CAD build for the part. Positions are in the model's coordinates, mm. Face numbers are marked on the shaded views. A direction names the side the tool comes from. Coordinates: 2 decimals unless noted, no trailing zeros. Loops run counter-clockwise (first coordinate to the right, second up) from the corner with the lowest first, then second, coordinate; pieces in that order, holes last. Notation, with made-up numbers: (82, -35) -> (125, -35) arc R9 ccw to (125, -24) -> close; hole circle Ø11 at (-9.75, 87.25). An arc over 180 degrees is marked (long way). Answer as a JSON object with one key per item and string values. Group by question number.
from build123d import *

# Parameters (mm, degrees)
SKETCH1_W           = 163
SKETCH1_H           = 113
OUTERCUT_DEPTH      = 23
FILLET2_R           = 2.5
FILLET3_R           = 2.5
SKETCH2_W           = 155
SKETCH2_H           = 105
INNERCUT_DEPTH      = 20
BOSS_EXTRUDE5_DEPTH = 3


with BuildPart() as part:
    # Sketch1 → OuterCut (new body)
    with BuildSketch(Plane(origin=(0, 0, 0), x_dir=(1, 0, 0), z_dir=(0, 1, 0))):
        Rectangle(SKETCH1_W, SKETCH1_H)
    extrude(amount=OUTERCUT_DEPTH)

    # Fillet2
    fillet2_edges = [part.edges().sort_by_distance(p)[0] for p in [
        (81.5, 11.5, 56.5),
    ]]
    fillet(fillet2_edges, radius=FILLET2_R)

    # Fillet3
    fillet3_edges = [part.edges().sort_by_distance(p)[0] for p in [
        (-81.5, 11.5, 56.5),
        (-81.5, 11.5, -56.5),
        (81.5, 11.5, -56.5),
    ]]
    fillet(fillet3_edges, radius=FILLET3_R)

    # Sketch2 → InnerCut (cut)
    with BuildSketch(Plane(origin=(0, 23, 0), x_dir=(1, 0, 0), z_dir=(0, 1, 0))):
        Rectangle(SKETCH2_W, SKETCH2_H)
    extrude(amount=-INNERCUT_DEPTH, mode=Mode.SUBTRACT)

    # Sketch9 → Boss-Extrude5 (add)
    with BuildSketch(Plane(origin=(0, 23, 0), x_dir=(1, 0, 0), z_dir=(0, 1, 0))):
        with BuildLine():
            Line((58.5, -53.7), (61.5, -53.7))
            ThreePointArc((61.5, -53.7), (62.3, -54.5), (61.5, -55.3))
            Line((61.5, -55.3), (58.5, -55.3))
            ThreePointArc((58.5, -55.3), (57.7, -54.5), (58.5, -53.7))
        make_face()
        with BuildLine():
            Line((-61.5, -53.7), (-58.5, -53.7))
            ThreePointArc((-58.5, -53.7), (-57.7, -54.5), (-58.5, -55.3))
            Line((-58.5, -55.3), (-61.5, -55.3))
            ThreePointArc((-61.5, -55.3), (-62.3, -54.5), (-61.5, -53.7))
        make_face()
        with BuildLine():
            Line((-61.5, 55.3), (-58.5, 55.3))
            ThreePointArc((-58.5, 55.3), (-57.7, 54.5), (-58.5, 53.7))
            Line((-58.5, 53.7), (-61.5, 53.7))
            ThreePointArc((-61.5, 53.7), (-62.3, 54.5), (-61.5, 55.3))
        make_face()
        with BuildLine():
            Line((58.5, 55.3), (61.5, 55.3))
            ThreePointArc((61.5, 55.3), (62.3, 54.5), (61.5, 53.7))
            Line((61.5, 53.7), (58.5, 53.7))
            ThreePointArc((58.5, 53.7), (57.7, 54.5), (58.5, 55.3))
        make_face()
    extrude(amount=BOSS_EXTRUDE5_DEPTH)


solid = part.part
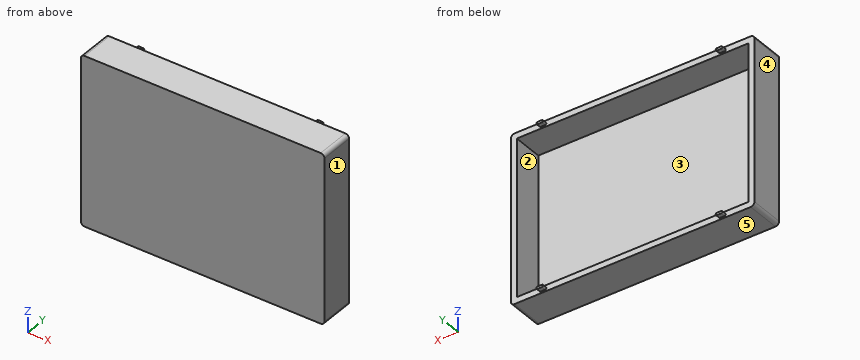
Item 1: Band-saw the part on B-B, the plane y = 17.5. List the corners of the cut face in (x, z).
Item 2: 3-axis set-ups, long thin cutter, end or side, ignore diameter. For the marked faces 1 and 2: which of +Z, -Z, +X, -X, +Y, -Y reach the whole face in a straight line?
Item 3: Flat gauge pins, fed straight in: P1, Ø3.5, axis at x = -60.5, y = 25, coming from the -Z side; P2, Ø1.5, axis at x = -10.5, z = -39.5, coming from the +Y side; P3, Ø0.9, axis at x = 60, y = 25, coming from the +Z side. Where does each tip first touch, or does it go through?
Item 4: Band-saw the part on C-C, the plane x = -7.5. List the corners of the cut face in (y, z), and give its area (3 significant figures).
Item 5: Band-saw the part on A-A, the plane z = 44.5. List the corners of the cut face in (x, y).
Item 6: Pull direction Z, two halves, no side cores. Call the marked faces 3, 4 and 5: +Z half, -Z half, draft (parallel to the pull), parting line (faces both ways), or undercut.
Item 7: Drill centre lines: L1, parallel to Z at x = 43, y = 9.5; L2, parallel to X at y = 14, z = 42; L3, parallel to Y at x = 20, z = -41. Where is each one in solid material? Low to high.
Reply:
{
 "1": {"outline": "(-81.5, -54) arc R2.5 ccw to (-79, -56.5) -> (79, -56.5) arc R2.5 ccw to (81.5, -54) -> (81.5, 54) arc R2.5 ccw to (79, 56.5) -> (-79, 56.5) arc R2.5 ccw to (-81.5, 54) -> close; hole (-77.5, -52.5) -> (77.5, -52.5) -> (77.5, 52.5) -> (-77.5, 52.5) -> close"},
 "2": {"face 1": "+Z, -Z, +X, +Y, -Y", "face 2": "+Y"},
 "3": {"P1": "z = -55.3", "P2": "y = 3", "P3": "z = 55.3"},
 "4": {"outline": "(0, -56.5) -> (23, -56.5) -> (23, -52.5) -> (3, -52.5) -> (3, 52.5) -> (23, 52.5) -> (23, 56.5) -> (0, 56.5) -> close", "area": "499 mm²"},
 "5": {"outline": "(-81.5, 0) -> (81.5, 0) -> (81.5, 23) -> (77.5, 23) -> (77.5, 3) -> (-77.5, 3) -> (-77.5, 23) -> (-81.5, 23) -> close"},
 "6": {"face 3": "undercut", "face 4": "draft", "face 5": "-Z half"},
 "7": {"L1": "-56.5 to -52.5, 52.5 to 56.5", "L2": "-81.5 to -77.5, 77.5 to 81.5", "L3": "0 to 3"}
}
